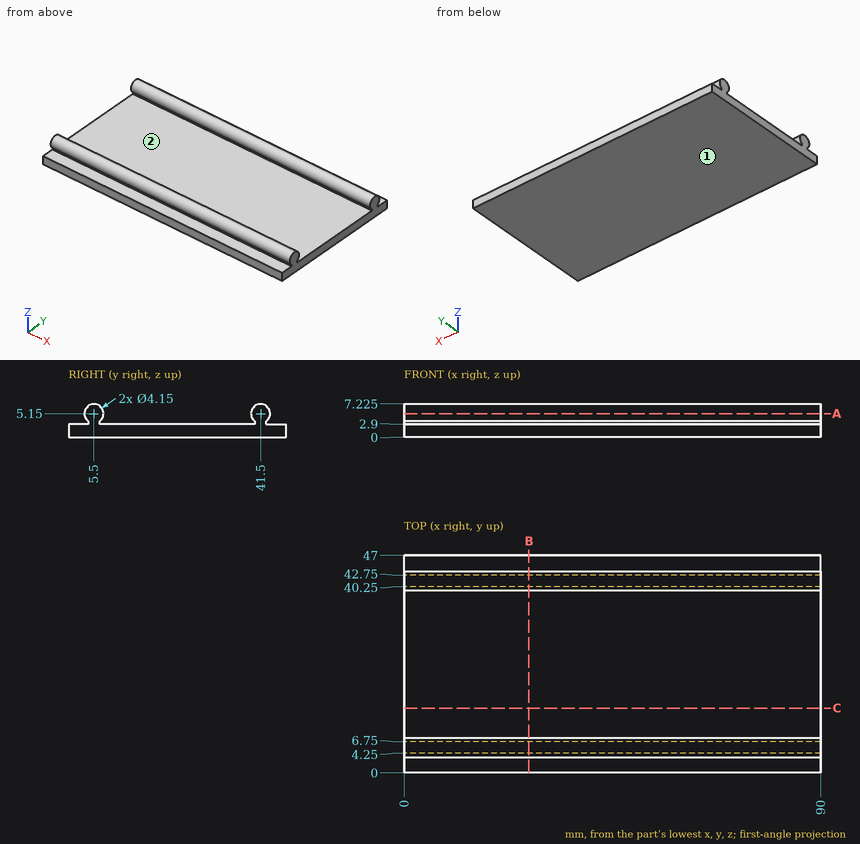
Geometry: see drawing. Coordinates: mm, zero at the bounding-box minimum. Coordinates: 2 decimals unless noted, no trailing zeros. Order: outer loops, then holes, each group sorted by start corner. A loop starts at its lowest first (then second) coordinate and runs counter-clockwise, first axis right, second up. Notation, with made-up numbers: M 43,74 L 79,74 A27 cw 79,100 Z; hole C -10,83.25 d8. An arc over 180 degrees is marked long. Write item = value, one per line. Start each with the question number.
(1) Section A-A on z = 5.15. Output: boundary loops of the cut face in (x, y) (3 decimals).
(2) Pull-direction query (Y, two-part tool) for the marked faces 1 and 2; classes: released by +Y, released by -Y, zero draft, split by the parting line, or undercut.
(3) Section B-B on x = 27. Output: boundary loops of the cut face in (y, z) (3 decimals), and give its area (3 significant figures).
(4) First-contact query: P1, Ø1, axis at x = 70.5, z = 3.5, coming from the +Y side; P2, Ø3.5, axis at x = 30, y = 2.5, coming from the +Z side; P3, Ø0.5, axis at x = 65.5, z = 3.5, coming from the -Y side. Flat tips, straight axial feed; report the tip coordinate or a pass-through.
(5) Line query: line 1 along Z through (x, y) = (25, 23); line 2 along Y through (x, z) = (59.5, 5.25); line 3 along Z through (x, y) = (39, 43). Output: solid intervals per line, ascending. Write a range as [from, to].
(6) Section C-C on y = 14. Output: boundary loops of the cut face in (x, z).
Result set:
q1.outline = M 0,3.425 L 90,3.425 L 90,7.575 L 0,7.575 Z; M 0,39.425 L 90,39.425 L 90,43.575 L 0,43.575 Z
q2.face_1 = zero draft
q2.face_2 = undercut
q3.outline = M 0,0 L 47,0 L 47,2.9 L 42.75,2.9 L 42.75,3.494 A2.075 ccw long 40.25,3.494 L 40.25,2.9 L 6.75,2.9 L 6.75,3.494 A2.075 ccw long 4.25,3.494 L 4.25,2.9 L 0,2.9 Z
q3.area = 165 mm²
q4.P1 = 43.23
q4.P2 = 6.81
q4.P3 = 3.97
q5.line_1 = [0, 2.9]
q5.line_2 = [3.43, 7.57], [39.43, 43.57]
q5.line_3 = [0, 2.9], [3.72, 6.58]
q6.outline = M 0,0 L 90,0 L 90,2.9 L 0,2.9 Z
